Part model, mm, in its own coordinate system. Face numbers are marked on the shaded views. A direction names the side the tool comes from. Coordinates: 2 decimals unless noted, no trailing zeros. Loops run counter-clockwise (first coordinate to the right, second up) from the corner with the lowest first, then second, coordinate; pieces in that order, holes last. Notation, with made-up numbers: M -7,55 L 34,55 A34 ccw 34,87 Z; hole C 22.25,55.5 d6. An arc over 180 degrees is marked long. Use a Markdown table: item, result. Add a question column.
1) Tool access for the marked faces 5, 6 and 7: list every direction of +Z, -Z, +X, -X, +Y, -Y with a clear straight run to the whole face (end or side of a thin tool).
2) Band-saw the part on C-C (y = 83). List the corners of the cut face in (x, z), plus the area to 3 significant figures.
3) Wall check: probe 1 along X at (y, z) = (-26.5, 24.5); probe 2 along Y at (x, z) = (-22.5, 48.5); probe 3 along X at (y, z) = (66, 73.5). Give the ranges that are in metal, low to high. Write a range as from..to.
4) Band-saw the part on D-D (z = 20). List the corners of the cut face in (x, y).
5) Pin check, flat tips, straight feed: pin 1 Ø5 at (x, y) = (-40.5, 48.5) entering from -Z; pin 2 Ø9.5 at (y, z) = (-19.5, 17.5) entering from +X; pin 3 Ø8 at (x, z) = (-45, 48) entering from -Y; pin 4 Ø8 at (x, z) = (-25.5, 39) entering from +Y. Stop position of each tip, or through.
6) Pull direction Y, two halves, no side cores. Call the marked faces 1, 2, 3 and 4: released by +Y, released by -Y, zero draft, split by the parting line, or undercut.
7) Band-saw the part on A-A (z = 60). List the corners of the cut face in (x, y).
8) Band-saw the part on B-B (x = -9). List the corners of the cut face in (y, z), plus the area to 3 significant figures.
from build123d import *

# Parameters (mm, degrees)
IZIM1_R                     = 25
IZIM1_R_2                   = 15
Y_KSEKLIK_EKSTR_ZYON1_DEPTH = 80
IZIM3_W                     = 26
IZIM3_H                     = 32
Y_KSEKLIK_EKSTR_ZYON3_DEPTH = 40
RADYUS2_RADIUS              = 20
RADYUS2_LENGTH              = 26
IZIM5_W                     = 6
IZIM5_H                     = 44.006307857
KES_EKSTR_ZYON1_DEPTH       = 107.133079222
KES_EKSTR_ZYON2_DEPTH       = 100.800958853
KES_EKSTR_ZYON2_DEPTH_BACK  = 100.800958853
IZIM7_R                     = 10
IZIM9_W                     = 20
IZIM9_H                     = 32
Y_KSEKLIK_EKSTR_ZYON4_DEPTH = 40
Y_KSEKLIK_EKSTR_ZYON5_DEPTH = 5
IZIM11_R                    = 20
IZIM11_R_2                  = 12.5
Y_KSEKLIK_EKSTR_ZYON6_DEPTH = 20
KES_EKSTR_ZYON3_DEPTH       = 130.453305469
KES_EKSTR_ZYON3_DEPTH_BACK  = 130.453305469
IZIM12_R                    = 12.5


with BuildPart() as part:
    # Çizim1 → Yükseklik-Ekstrüzyon1 (new body)
    with BuildSketch(Plane.XY):
        with Locations((-27.727849989, 20.650896384)):
            Circle(IZIM1_R)
        with Locations((-27.727849989, 20.650896384)):
            Circle(IZIM1_R_2, mode=Mode.SUBTRACT)
    extrude(amount=Y_KSEKLIK_EKSTR_ZYON1_DEPTH)

    # Çizim3 → Yükseklik-Ekstrüzyon3 (add)
    with BuildSketch(Plane(origin=(0, 0, 0), x_dir=(-1, 0, 0), z_dir=(0, 0, -1))):
        with Locations((28.149550203, -16.534219889)):
            Rectangle(IZIM3_W, IZIM3_H)
    extrude(amount=-Y_KSEKLIK_EKSTR_ZYON3_DEPTH)

    # Radyus2: full round fillet: the end face becomes a half cylinder, R = half its width
    radyus2_face = Plane((-28.149550203, -32.534219889, 20), x_dir=(-1, 0, 0), z_dir=(0, -1, 0))  # on the end face: x along it, z out of the body
    radyus2_slab = radyus2_face.offset(-RADYUS2_RADIUS / 2) * Box(RADYUS2_LENGTH, 2 * RADYUS2_RADIUS, RADYUS2_RADIUS, mode=Mode.PRIVATE)  # the body's end, R deep
    radyus2_round = Plane((-28.149550203, -12.534219889, 20), x_dir=(0, -1, 0), z_dir=(-1, 0, 0)) * Cylinder(RADYUS2_RADIUS, RADYUS2_LENGTH, mode=Mode.PRIVATE)  # its axis R under the face
    add(radyus2_slab - radyus2_round, mode=Mode.SUBTRACT)

    # Çizim5 → Kes-Ekstrüzyon1 (cut, through all)
    with BuildSketch(Plane(origin=(0, 0, 0), x_dir=(-1, 0, 0), z_dir=(0, 0, -1))):
        with Locations((28.149550203, -10.53106596)):
            Rectangle(IZIM5_W, IZIM5_H)
    extrude(amount=-KES_EKSTR_ZYON1_DEPTH, mode=Mode.SUBTRACT)

    # Çizim7 → Kes-Ekstrüzyon2 (cut, two sides: drawn at the far end of the back side and taken through both)
    with BuildSketch(Plane.ZY.offset(41.149550203).offset(-KES_EKSTR_ZYON2_DEPTH_BACK)):
        with Locations(Location((20, -12.534219889, 0), (0, 0, 90))):
            Circle(IZIM7_R)
    extrude(amount=KES_EKSTR_ZYON2_DEPTH + KES_EKSTR_ZYON2_DEPTH_BACK, mode=Mode.SUBTRACT)

    # Çizim9 → Yükseklik-Ekstrüzyon4 (add)
    with BuildSketch(Plane.XY.offset(80)):
        with Locations((-27.673094682, 59.587594228)):
            Rectangle(IZIM9_W, IZIM9_H)
    extrude(amount=-Y_KSEKLIK_EKSTR_ZYON4_DEPTH)

    # Çizim10 → Yükseklik-Ekstrüzyon5 (add, symmetric)
    with BuildSketch(Plane.ZY.offset(27.673094682)):
        Polygon((0, 45.650896384), (40, 63.587594228), (40, 45.639566476), align=None)
    extrude(amount=Y_KSEKLIK_EKSTR_ZYON5_DEPTH, both=True)

    # Çizim11 → Yükseklik-Ekstrüzyon6 (add, symmetric)
    with BuildSketch(Plane.ZY.offset(27.673094682)):
        with Locations((60, 75.587594228)):
            Circle(IZIM11_R)
        with Locations((60, 75.587594228)):
            Circle(IZIM11_R_2, mode=Mode.SUBTRACT)
    extrude(amount=Y_KSEKLIK_EKSTR_ZYON6_DEPTH, both=True)

    # Çizim12 → Kes-Ekstrüzyon3 (cut, two sides: drawn at the far end of the back side and taken through both)
    with BuildSketch(Plane.ZY.offset(37.673094682).offset(-KES_EKSTR_ZYON3_DEPTH_BACK)):
        with Locations((60, 75.587594228)):
            Circle(IZIM12_R)
    extrude(amount=KES_EKSTR_ZYON3_DEPTH + KES_EKSTR_ZYON3_DEPTH_BACK, mode=Mode.SUBTRACT)


solid = part.part
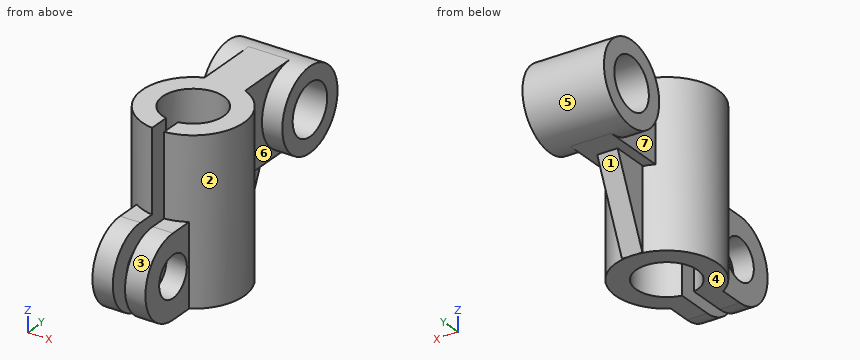
Entries:
| question | item | result |
|---|---|---|
| 1 | face 5 | none |
| 1 | face 6 | +X |
| 1 | face 7 | -X |
| 2 | outline | M -47.67,41.42 L -7.67,41.42 L -7.67,49.93 L -47.67,49.93 Z; M -47.67,70.07 L -7.67,70.07 L -7.67,78.58 L -47.67,78.58 Z |
| 2 | area | 681 mm2 |
| 3 | probe 1 | -41.15..-31.15, -25.15..-15.15 |
| 3 | probe 2 | -3.8..6.59, 34.71..70.69, 80.49..91.95 |
| 3 | probe 3 | -47.67..-7.67 |
| 4 | outline | M -41.15,-32.53 L -31.15,-32.53 L -31.15,-22.53 L -41.15,-22.53 Z; M -41.15,-2.53 L -31.15,-2.53 L -31.15,6.05 A15 cw long -25.15,5.87 L -25.15,-2.53 L -15.15,-2.53 L -15.15,-0.95 A25 ccw -27.2,45.65 L -22.67,45.65 L -22.67,54.62 L -32.67,54.62 L -32.67,45.65 L -28.26,45.65 A25 ccw -41,-0.53 L -41.15,-0.53 Z; M -25.15,-32.53 L -15.15,-32.53 L -15.15,-22.53 L -25.15,-22.53 Z |
| 5 | pin 1 | through |
| 5 | pin 2 | x = -15.15 |
| 5 | pin 3 | y = -0.54 |
| 5 | pin 4 | y = 86.12 |
| 6 | face 1 | released by +Y |
| 6 | face 2 | undercut |
| 6 | face 3 | released by -Y |
| 6 | face 4 | zero draft |
| 7 | outline | M -47.67,55.59 L -37.67,55.59 L -37.67,43.59 A25 ccw -31.15,-4.11 L -31.15,6.05 A15 cw long -25.15,5.87 L -25.15,-4.22 A25 ccw -17.78,43.59 L -17.67,43.59 L -17.67,55.59 L -7.67,55.59 L -7.67,63.09 L -47.67,63.09 Z; M -47.67,88.09 L -7.67,88.09 L -7.67,95.59 L -47.67,95.59 Z |
| 8 | outline | M 4.09,0 L 37.21,0 L 37.21,80 L 4.09,80 Z; C 75.59,60 d40; hole C 75.59,60 d25 |
| 8 | area | 3,420 mm2 |
